Input: part model. Units: mm. Frame: model coordinates. Give positions to 0.01 mm unless a question says otherwise; leave off trailing zeros. Loops run counter-clockwise (first coordinate to the right, second up) from the corner with the lowest first, then second, coordinate; pieces in that order, holes last. Notation, with made-up numbers: M -15,87.5 L 36,87.5 A5 cw 36,96.5 Z; hole C 13,22 d6. An arc over 180 degrees is marked long. Answer as a JSON object with one key per item and string values. Group by question number.
1) Ray query, L1, parallel to Z at x = 0, y = 8; L2, parallel to Z at x = 2, y = 12; L3, parallel to Z at x = 7, y = 35. Return the intervals inside material, ascending.
2) Draft query along Z for faces 1 (the flat face through (0.1, 12.7, 19.4)), 2 (the cylindrical face through (2.435, 9.658, -0.767)), 3 (the cylindrical face through (-15.218, 6.439, 11.669)). Return one class per face: +Z half, -Z half, draft (parallel to the pull), parting line (faces both ways), or undercut.
3) Section query A-A on y = 50.5. Return loops of the section in (x, z), plus the area to 3 significant figures.
4) Section query B-B on y = 74.5. Return loops of the section in (x, z), plus the area to 3 significant figures.
5) First-contact query: P1, Ø10, axis at y = 127.5, z = 1.5, coming from the +X side; P2, Ø10, axis at y = 144.5, z = 4, coming from the +X side; P3, Ø8, axis at y = 61.5, z = 0.5, coming from the -X side. Flat tips, straight axial feed; report the tip coordinate or a pass-through.
from build123d import *

# Parameters (mm, degrees)
TAP_DRILL_FOR_1_4_20_TAP1_D     = 5.1054
TAP_DRILL_FOR_1_4_20_TAP1_DEPTH = 19.05
TAP_DRILL_FOR_1_4_20_TAP1_TIP   = 1.533816902


with BuildPart() as part:
    # Sketch2 → Revolve1 (revolve)
    with BuildSketch(Plane.XY):
        with BuildLine():
            Line((21.9329, 12.7), (1.257640447, 159.812115824))
            ThreePointArc((1.257640447, 159.812115824), (0.833194967, 160.593847152), (0, 160.905365985))
            Line((0, 160.905365985), (0, 0))
            Line((0, 0), (19.177, 0))
            Line((19.177, 0), (19.177, 12.7))
            Line((19.177, 12.7), (21.9329, 12.7))
        make_face()
    revolve(axis=Axis((0, 0, 0), (0, 1, 0)))

    # Tap Drill for 1/4-20 Tap1
    with Locations(Plane(origin=(0, 0, 0), x_dir=(-1, 0, 0), z_dir=(0, -1, 0))):
        with Locations((0, 0)):
            Hole(TAP_DRILL_FOR_1_4_20_TAP1_D / 2, depth=TAP_DRILL_FOR_1_4_20_TAP1_DEPTH)
            with Locations((0, 0, -(TAP_DRILL_FOR_1_4_20_TAP1_DEPTH + TAP_DRILL_FOR_1_4_20_TAP1_TIP / 2))):  # 118° drill point
                Cone(0, TAP_DRILL_FOR_1_4_20_TAP1_D / 2, TAP_DRILL_FOR_1_4_20_TAP1_TIP, mode=Mode.SUBTRACT)


solid = part.part
Output:
{
 "1": {"L1": "z = -19.18 to -2.55, 2.55 to 19.18", "L2": "z = -19.07 to -1.59, 1.59 to 19.07", "L3": "z = -17.45 to 17.45"},
 "2": {"face 1": "draft", "face 2": "undercut", "face 3": "parting line"},
 "3": {"outline": "C 0,0 d33.24", "area": "868 mm^2"},
 "4": {"outline": "C 0,0 d26.49", "area": "551 mm^2"},
 "5": {"P1": "stops at x = 6.47", "P2": "stops at x = 3.88", "P3": "stops at x = -15.63"}
}
